from build123d import *

# Parameters (mm, degrees)
F1_DEPTH = 7.5
F2_R     = 5
F3_DEPTH = 25
F4_SIZE  = 5
F5_R     = 2


with BuildPart() as f1:
    # F0 (on Front) → F1 (new body, symmetric)
    with BuildSketch(Plane.XZ):
        Polygon((0, -33.556624), (0, 0), (5.1, 2.944486), (5.1, 69.387862), (2.6, 69.387862), (2.6, 4.387862), (-2.5, 1.443376), (-2.5, -33.556624), align=None)
    extrude(amount=F1_DEPTH, both=True)

    # F2 (on face) → F3 (cut)
    with BuildSketch(Plane(origin=(2.6, 0, 0), x_dir=(0, -1, 0), z_dir=(-1, 0, 0))):
        with BuildLine():
            Line((-7.5, 69.387862), (-7.5, 61.887862))
            ThreePointArc((-7.5, 61.887862), (-5.303301, 67.191163), (0, 69.387862))
            Line((0, 69.387862), (-7.5, 69.387862))
        make_face()
        with Locations((0, 62.387862)):
            Circle(F2_R)
        with BuildLine():
            Line((7.5, 69.387862), (0, 69.387862))
            ThreePointArc((0, 69.387862), (5.303301, 67.191163), (7.5, 61.887862))
            Line((7.5, 61.887862), (7.5, 69.387862))
        make_face()
    extrude(amount=-F3_DEPTH, mode=Mode.SUBTRACT)

    # F4
    f4_edges = [f1.edges().sort_by_distance(p)[0] for p in [
        (-1.25, 7.5, -33.556624),
        (-1.25, -7.5, -33.556624),
    ]]
    chamfer(f4_edges, length=F4_SIZE)

    # F5
    f5_edges = [f1.edges().sort_by_distance(p)[0] for p in [
        (-2.5, 0, 1.443376),
        (2.6, 0, 4.387862),
        (5.1, 0, 2.944486),
        (0, 0, 0),
    ]]
    fillet(f5_edges, radius=F5_R)


solid = f1.part
Can you work these out from the model? Positions are in its coordinate system, mm. A direction names the side the tool comes from. Coordinates: 2 decimals unless noted, no trailing zeros. Order: outer loops, then holes, each group sorted by start corner. A loop starts at its lowest first (then second) coordinate and runs counter-clockwise, first axis right, second up. Notation, with made-up numbers: M 47,-7.5 L 79,-7.5 A17 ccw 79,11.5 Z; hole C -6,-23.5 d9. An arc over 180 degrees is marked long. Answer as CSV lines item,"result".
(1) Please list where these lines run through material, in increasing order: L1, parallel to X at y = -1.75, z = 28; L2, parallel to Z at x = 2.75, y = -1.5; L3, parallel to X at y = -7, z = -3.5.
Geometry check:
L1,"2.6 to 5.1"
L2,"1.59 to 57.62, 67.16 to 69.24"
L3,"-2.5 to 0"
(2) I'm going to push flat-ended pins straight in: pin 1 (4.5 mm diameter, centred on y = 1, z = 32.5, fed in from -X); pin 2 (1 mm diameter, centred on y = 0, z = 1.5, fed in from +X); pin 3 (1.5 mm diameter, centred on x = 0.5, y = 4.5, fed in from +Z). Where does each tip first touch, or does it pass through?
Geometry check:
pin 1,"x = 2.6"
pin 2,"x = 3.46"
pin 3,"z = 3.61"
(3) On a 3-axis mill with a long thin cutter (end or side, diameter ignored), from which of +Z, -Z, +X, -X, +Y, -Y can I reach the whole of each face in a straight line? I mean faces 1 (the flat face through (2.6, 0, 38)), 2 (the flat face through (0, 0, -18)), 3 (the flat face through (-2.5, 0, -16)). Say none if no direction works.
Geometry check:
face 1,"+Z, -X, +Y, -Y"
face 2,"-Z, +X, +Y, -Y"
face 3,"+Z, -Z, -X, +Y, -Y"
(4) If we mould it in two halves opening along Y, with no side actions, what happens to faces 4 (the cylindrical face through (3.832, 1.084, 57.507)), 5 (the flat face through (5.1, 0, 36)), 6 (the flat face through (3, 7.5, 17))? For each: released by +Y, released by -Y, zero draft, split by the parting line, or undercut.
Geometry check:
face 4,"undercut"
face 5,"zero draft"
face 6,"released by +Y"
(5) Suppose I cut it at A-A on y = -4. Please give me the cut outline in (x, z).
Geometry check:
outline,"M -2.5,-32.06 L 0,-32.06 L 0,-1.15 A2 cw 1,0.58 L 4.1,2.37 A2 ccw 5.1,4.1 L 5.1,59.39 L 2.6,59.39 L 2.6,5.54 A2 cw 1.6,3.81 L -1.5,2.02 A2 ccw -2.5,0.29 Z; M 2.6,65.39 L 5.1,65.39 L 5.1,68.23 L 2.6,68.23 Z"
(6) Suppose I cut it at B-B on z = 53. Please give me the cut outline in (x, y), plus the area to 3 significant figures.
Geometry check:
outline,"M 2.6,-7.5 L 5.1,-7.5 L 5.1,7.5 L 2.6,7.5 Z"
area,"37.5 mm^2"
